from build123d import *

# Parameters (mm, degrees)
F1_DEPTH = 20.32
F2_R     = 0.762


with BuildPart() as f1:
    # F0 (on Front) → F1 (new body)
    with BuildSketch(Plane.XZ):
        with BuildLine():
            ThreePointArc((21.306762, 16.25961), (-4.560012, 9.701865), (-31.242051, 10.105342))
            ThreePointArc((-31.242051, 10.105342), (-37.051563, 5.452601), (-31.985246, 0))
            ThreePointArc((-31.985246, 0), (-5.531263, -3.5044), (19.097811, -13.77585))
            ThreePointArc((19.097811, -13.77585), (21.956659, -15.206004), (24.972497, -16.265755))
            Line((24.972497, -16.265755), (37.195468, -19.713795))
            Line((37.195468, -19.713795), (38.145715, -16.34526))
            Line((38.145715, -16.34526), (25.922744, -12.89722))
            ThreePointArc((25.922744, -12.89722), (23.322474, -11.983497), (20.857562, -10.750412))
            ThreePointArc((20.857562, -10.750412), (-4.619955, -0.125122), (-31.985246, 3.5))
            ThreePointArc((-31.985246, 3.5), (-33.56099, 5.195888), (-31.754095, 6.643))
            ThreePointArc((-31.754095, 6.643), (-4.152891, 6.225624), (22.604963, 13.009276))
            ThreePointArc((22.604963, 13.009276), (25.223752, 13.868481), (27.92972, 14.391958))
            Line((27.92972, 14.391958), (40.52562, 16.014699))
            Line((40.52562, 16.014699), (40.078408, 19.486011))
            Line((40.078408, 19.486011), (27.482508, 17.863269))
            ThreePointArc((27.482508, 17.863269), (24.344079, 17.256131), (21.306762, 16.25961))
        make_face()
    extrude(amount=F1_DEPTH)

    # F2
    f2_edges = [f1.edges().sort_by_distance(p)[0] for p in [
        (33.780458, -20.32, 18.67464),
        (24.344079, -20.32, 17.256131),
        (-4.560012, -20.32, 9.701865),
        (-37.051563, -20.32, 5.452601),
        (-5.531263, -20.32, -3.5044),
        (21.956659, -20.32, -15.206004),
        (31.083982, -20.32, -17.989775),
        (37.670591, -20.32, -18.029527),
        (32.034229, -20.32, -14.62124),
        (23.322474, -20.32, -11.983497),
        (-4.619955, -20.32, -0.125122),
        (-33.56099, -20.32, 5.195888),
        (-4.152891, -20.32, 6.225624),
        (25.223752, -20.32, 13.868481),
        (34.22767, -20.32, 15.203329),
        (40.302014, -20.32, 17.750355),
        (33.780458, 0, 18.67464),
        (24.344079, 0, 17.256131),
        (-4.560012, 0, 9.701865),
        (-37.051563, 0, 5.452601),
        (-5.531263, 0, -3.5044),
        (21.956659, 0, -15.206004),
        (31.083982, 0, -17.989775),
        (37.670591, 0, -18.029527),
        (32.034229, 0, -14.62124),
        (23.322474, 0, -11.983497),
        (-4.619955, 0, -0.125122),
        (-33.56099, 0, 5.195888),
        (-4.152891, 0, 6.225624),
        (25.223752, 0, 13.868481),
        (34.22767, 0, 15.203329),
        (40.302014, 0, 17.750355),
        (40.52562, -10.16, 16.014699),
        (40.078408, -10.16, 19.486011),
        (37.195468, -10.16, -19.713795),
        (38.145715, -10.16, -16.34526),
    ]]
    fillet(f2_edges, radius=F2_R)


solid = f1.part
Geometry check sheet. Reference: the model listing, model coordinates, mm. A direction names the side the tool comes from. Coordinates: 2 decimals unless noted, no trailing zeros. Order: outer loops, then holes, each group sorted by start corner. A loop starts at its lowest first (then second) coordinate and runs counter-clockwise, first axis right, second up. Notation, with made-up numbers: (-25, 71.25) -> (-5, 71.25) arc R13 ccw to (-5, 95.25) -> close; hole circle Ø6 at (67.5, -8). An arc over 180 degrees is marked (long way). Use a Markdown table: item, result. Add a question column.
1. Material ranges on L1, parallel to Z at x = 15, y = -9; L2, parallel to Z at x = -22.5, y = -9.5; L3, parallel to Y at x = 31.5, z = 15.5, recorded low to high.
2. Go/stop test with flat-tipped pins: pin 1 Ø5 at (y, z) = (-9, 8.5) entering from -X; pin 2 Ø1 at (x, y) = (-26, -14) entering from -Z; pin 3 Ø12 at (x, y) = (-21, -9) entering from -Z. Record where each tip stops, or that it passes through.
3. Mould release check, pull along Z, two halves, no side actions. Record for faces 4 (the face through (33.9, -20.09, 15.38)), 5 (the face through (37.667, -10.028, -18.043)), 6 (the face through (33.485, -10.028, 18.637)): pulls with the +Z half, pulls with the -Z half, needs draft (parallel to the pull), parting line crosses it, or undercut.
4. Set-up check for faces 1 (the face through (31.528, -20.091, -14.704)), 2 (the face through (33.9, -0.23, 15.38)), 3 (the face through (23.36, -10.03, -12)): record each of +Z, -Z, +X, -X, +Y, -Y from which the full face is reachable in a straight line by a thin tool's end or side.
5. Cross-section at A-A (y = -6.25). Enter the section's corners in (x, z).
Filled sheet:
| question | item | result |
|---|---|---|
| 1 | L1 | -11.52 to -7.59, 10.31 to 13.98 |
| 1 | L2 | -0.44 to 3.07, 5.69 to 9.2 |
| 1 | L3 | -20.31 to -0.01 |
| 2 | pin 1 | x = -36.98 |
| 2 | pin 2 | z = -0.21 |
| 2 | pin 3 | z = -1.43 |
| 3 | face 4 | undercut |
| 3 | face 5 | pulls with the -Z half |
| 3 | face 6 | pulls with the +Z half |
| 4 | face 1 | +X, -Y |
| 4 | face 2 | +X, +Y |
| 4 | face 3 | +X, +Y, -Y |
| 5 | outline | (-31.99, 0) arc R101.6 cw to (19.1, -13.78) arc R25.4 ccw to (24.97, -16.27) -> (36.46, -19.51) arc R0.76 ccw to (37.4, -18.98) -> (37.94, -17.08) arc R0.76 ccw to (37.41, -16.14) -> (25.92, -12.9) arc R21.9 cw to (20.86, -10.75) arc R105.1 ccw to (-31.99, 3.5) arc R1.58 cw (long way) to (-31.75, 6.64) arc R105.1 ccw to (22.6, 13.01) arc R21.9 cw to (27.93, 14.39) -> (39.77, 15.92) arc R0.76 ccw to (40.43, 16.77) -> (40.18, 18.73) arc R0.76 ccw to (39.32, 19.39) -> (27.48, 17.86) arc R25.4 ccw to (21.31, 16.26) arc R101.6 cw to (-31.24, 10.11) arc R5.08 ccw (long way) to start |
